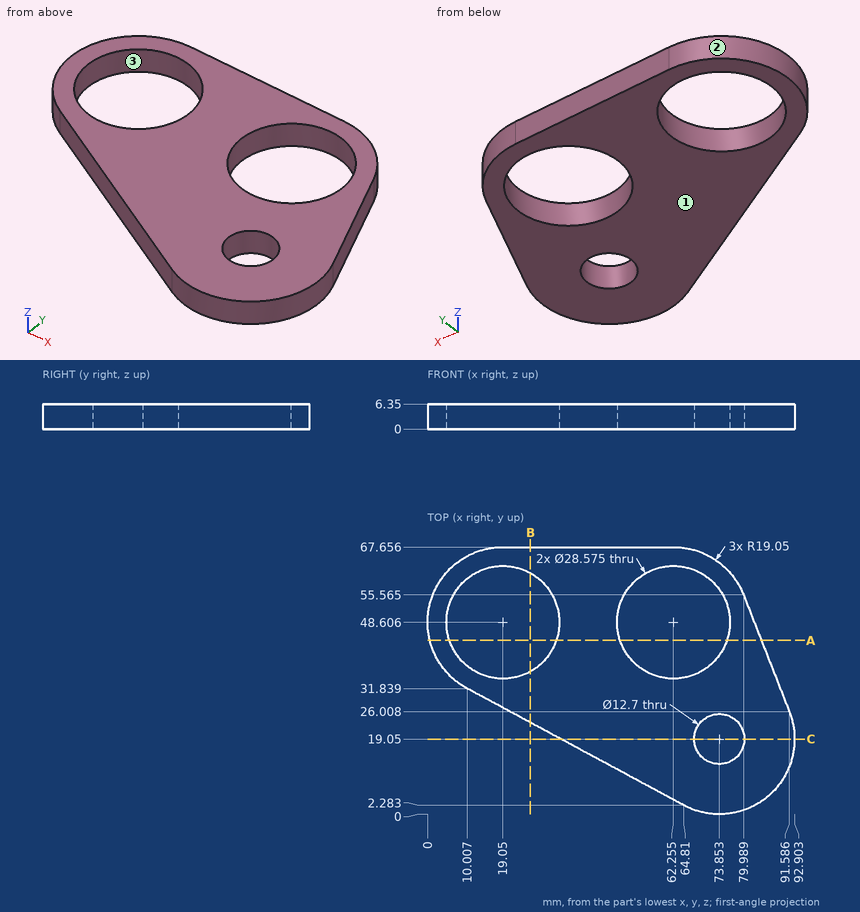
Can you work these out from the drawing? Everything is in mm from the part's minimum corner. Coordinates: 2 decimals unless noted, no trailing zeros. Loops run counter-clockwise (first coordinate to the right, second up) from the corner with the lowest first, then second, coordinate; pieces in that order, holes last.
1) For pin 1 (1.5 mm diameter, centred on y = 27, z = 5.5, fed in from +X); pin 2 (2 mm diameter, centred on y = 28.5, z = 1.5, fed in from -X) (1 decimal); pin 3 (2 mm diameter, centred on y = 42.5, z = 3, fed in from +X), each with a flat end and sliding along its axis, tell me the tip position at first contact or that it passes through.
2) Imagine slicing it at B-B on x = 26. List the corners of the cut face in (y, z) for me.
3) Imagine slicing it at A-A on y = 44. State how many separate pieces and enclosed holes the cut face has, plus the area to 3 significant figures.
4) Thinking about a two-plate mould opening in X: for the marked faces 1, 2 and 3, which applies, pulls with the +X half, pulls with the -X half, needs draft (parallel to the pull), parting line crosses it, or undercut?
5) I need wall thicknesses on probe 1 along X at (y, z) = (56.5, 1.5) (1 decimal); probe 2 along X at (y, z) = (44.5, 6) (1 decimal); probe 3 along Y at (x, z) = (62, 1.5) (1 decimal). Which ranges of each line are inside material? Lowest first, please.
6) Imagine slicing it at C-C on y = 19.05. List the corners of the cut face in (x, z) for me, plus the area to 3 significant figures.
Completed:
1. pin 1: stops at x = 91.49
1. pin 2: stops at x = 14.3
1. pin 3: stops at x = 85.51
2. outline: (23.21, 0) - (36.12, 0) - (36.12, 6.35) - (23.21, 6.35) - close; (61.09, 0) - (67.66, 0) - (67.66, 6.35) - (61.09, 6.35) - close
3. separate pieces: 3
3. enclosed holes: 0
3. area: 190 mm2
4. face 1: needs draft
4. face 2: pulls with the -X half
4. face 3: undercut
5. probe 1: x = 1.7 to 7.1, 31 to 50.3, 74.2 to 79.6
5. probe 2: x = 0.4 to 5.4, 32.7 to 48.6, 75.9 to 84.3
5. probe 3: y = 3.8 to 34.3, 62.9 to 67.7
6. outline: (33.72, 0) - (67.5, 0) - (67.5, 6.35) - (33.72, 6.35) - close; (80.2, 0) - (92.9, 0) - (92.9, 6.35) - (80.2, 6.35) - close
6. area: 295 mm2
